Here's the drawing with two shaded views (mm, measured from the low corner). I have some questions. A direction names the side the tool comes from. Round coordinates to 2 decimals unless told otherwise and drop trailing zeros. Order: outer loops, then holes, each group sorted by start corner. A loop starts at its lowest first (then second) coordinate and runs counter-clockwise, first axis right, second up.
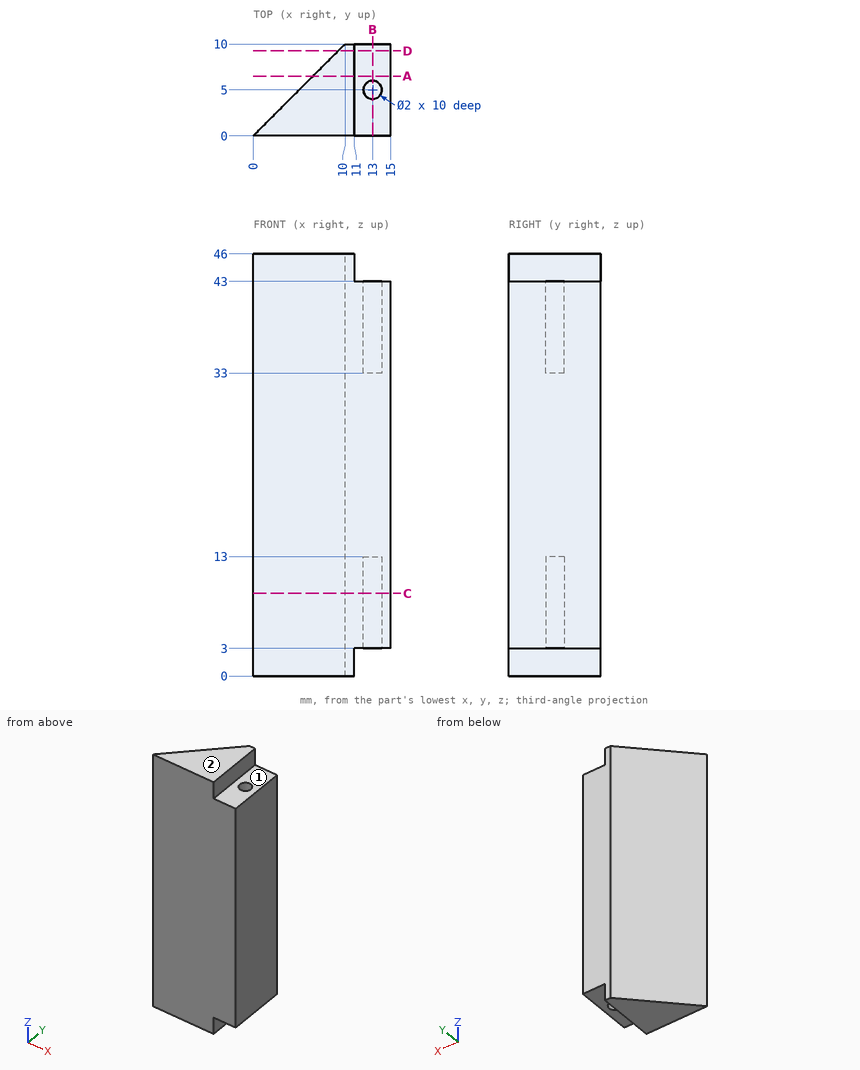
1. On a 3-axis mill with a long thin cutter (end or side, diameter ignored), from which of +Z, -Z, +X, -X, +Y, -Y can I reach the whole of each face in a straight line? I mean the marked faces 1 and 2. Say none if no direction works.
Evaluation:
face 1: +Z, +X, +Y, -Y
face 2: +Z, +X, -X, +Y, -Y
2. I'm going to push flat-ended pins straight in: P1, Ø1, axis at x = 12.5, y = 4.5, coming from the -Z side; P2, Ø8, axis at x = 11, z = 33, coming from the -Y side; P3, Ø3, axis at y = 2, z = 38.5, coming from the -X side; P4, Ø2.5, axis at x = 13, y = 5, coming from the +Z side. Where does each tip first touch, or does it pass through?
Evaluation:
P1: stops at z = 3
P2: stops at y = 0
P3: stops at x = 0.5
P4: stops at z = 43
3. If we section it at C-C, the plane z = 9: Write out the boundary of the cut face in (x, y), and give its area (3 significant figures).
Evaluation:
outline: (0, 0) - (15, 0) - (15, 10) - (10, 10) - close; hole circle Ø2 at (13, 5)
area: 96.9 mm2
4. If we section it at B-B, the plane x = 13: Write out the boundary of the cut face in (y, z).
Evaluation:
outline: (0, 3) - (4, 3) - (4, 13) - (6, 13) - (6, 3) - (10, 3) - (10, 43) - (6, 43) - (6, 33) - (4, 33) - (4, 43) - (0, 43) - close
5. If we section it at D-D, the plane y = 9.25: Write out the boundary of the cut face in (x, z), and give its area (4 significant figures).
Evaluation:
outline: (9.25, 0) - (11, 0) - (11, 3) - (15, 3) - (15, 43) - (11, 43) - (11, 46) - (9.25, 46) - close
area: 240.5 mm2
6. I need wall thicknesses on probe 1 along Y at (x, z) = (13, 5); probe 2 along Z at (x, y) = (12.75, 1.5); probe 3 along X at (y, z) = (4.25, 11.5). Which ranges of each line are inside material? Lowest first, please.
Evaluation:
probe 1: y = 0 to 4, 6 to 10
probe 2: z = 3 to 43
probe 3: x = 4.25 to 12.34, 13.66 to 15
7. If we section it at A-A, the plane y = 6.5: Write out the boundary of the cut face in (x, z), and give its area (3 significant figures).
Evaluation:
outline: (6.5, 0) - (11, 0) - (11, 3) - (15, 3) - (15, 43) - (11, 43) - (11, 46) - (6.5, 46) - close
area: 367 mm2
